```python
from build123d import *

# Parameters (mm, degrees)
SKETCH1_W           = 100
SKETCH1_H           = 105
SKETCH1_R           = 1.1
BOSS_EXTRUDE1_DEPTH = 2.5
SKETCH3_R           = 4
SKETCH3_R_2         = 1.1
BOSS_EXTRUDE2_DEPTH = 2.5
CHAMFER1_SIZE       = 1.25
SKETCH2_R           = 4.6
CUT_EXTRUDE1_DEPTH  = 0.6
SKETCH11_W          = 2.5
SKETCH11_H          = 2.5
BOSS_EXTRUDE5_DEPTH = 2.5


with BuildPart() as part:
    # Sketch1 → Boss-Extrude1 (new body)
    with BuildSketch(Plane(origin=(0, 0, 0), x_dir=(1, 0, 0), z_dir=(0, 1, 0))):
        Rectangle(SKETCH1_W, SKETCH1_H)
        with Locations(Location((-45, 45, 0), (0, 0, 270))):
            Circle(SKETCH1_R, mode=Mode.SUBTRACT)
        with Locations(Location((45, 45, 0), (0, 0, 90))):
            Circle(SKETCH1_R, mode=Mode.SUBTRACT)
        with Locations(Location((45, -45, 0), (0, 0, 270))):
            Circle(SKETCH1_R, mode=Mode.SUBTRACT)
        with Locations(Location((-45, -45, 0), (0, 0, 90))):
            Circle(SKETCH1_R, mode=Mode.SUBTRACT)
        Polygon((-40, 47.5), (40, 47.5), (40, 40), (47.5, 40), (47.5, -40), (40, -40), (40, -47.5), (-40, -47.5), (-40, -40), (-47.5, -40), (-47.5, 40), (-40, 40), align=None, mode=Mode.SUBTRACT)
    extrude(amount=BOSS_EXTRUDE1_DEPTH)

    # Sketch3 → Boss-Extrude2 (add)
    with BuildSketch(Plane(origin=(0, 0, 0), x_dir=(1, 0, 0), z_dir=(0, 1, 0))):
        with BuildLine():
            Line((-42.828427125, 40), (-6.891439137, 4.063012013))
            ThreePointArc((-6.891439137, 4.063012013), (-7.39103626, 3.061467459), (-7.745966692, 2))
            Line((-7.745966692, 2), (-40.338668084, 2))
            Line((-40.338668084, 2), (-47.5, 2))
            Line((-47.5, 2), (-47.5, -2))
            Line((-47.5, -2), (-43.661317629, -2))
            Line((-43.661317629, -2), (-7.745966692, -2))
            ThreePointArc((-7.745966692, -2), (-7.39103626, -3.061467459), (-6.891439137, -4.063012013))
            Line((-6.891439137, -4.063012013), (-42.828427125, -40))
            Line((-42.828427125, -40), (-40, -42.828427125))
            Line((-40, -42.828427125), (-4.063012013, -6.891439137))
            ThreePointArc((-4.063012013, -6.891439137), (-3.061467459, -7.39103626), (-2, -7.745966692))
            Line((-2, -7.745966692), (-2, -43.661317629))
            Line((-2, -43.661317629), (-2, -47.5))
            Line((-2, -47.5), (2, -47.5))
            Line((2, -47.5), (2, -43.661317629))
            Line((2, -43.661317629), (2, -7.745966692))
            ThreePointArc((2, -7.745966692), (3.061467459, -7.39103626), (4.063012013, -6.891439137))
            Line((4.063012013, -6.891439137), (40, -42.828427125))
            Line((40, -42.828427125), (42.828427125, -40))
            Line((42.828427125, -40), (6.891439137, -4.063012013))
            ThreePointArc((6.891439137, -4.063012013), (7.39103626, -3.061467459), (7.745966692, -2))
            Line((7.745966692, -2), (40.338675227, -2))
            ThreePointArc((40.338675227, -2), (42, -2.6), (43.661324773, -2))
            Line((43.661324773, -2), (47.5, -2))
            Line((47.5, -2), (47.5, 2))
            Line((47.5, 2), (43.661324773, 2))
            ThreePointArc((43.661324773, 2), (42, 2.6), (40.338675227, 2))
            Line((40.338675227, 2), (7.745966692, 2))
            ThreePointArc((7.745966692, 2), (7.39103626, 3.061467459), (6.891439137, 4.063012013))
            Line((6.891439137, 4.063012013), (42.828427125, 40))
            Line((42.828427125, 40), (40, 42.828427125))
            Line((40, 42.828427125), (4.063012013, 6.891439137))
            ThreePointArc((4.063012013, 6.891439137), (3.061467459, 7.39103626), (2, 7.745966692))
            Line((2, 7.745966692), (2, 40.338675227))
            ThreePointArc((2, 40.338675227), (2.6, 42), (2, 43.661324773))
            Line((2, 43.661324773), (2, 47.5))
            Line((2, 47.5), (-2, 47.5))
            Line((-2, 47.5), (-2, 43.661324773))
            ThreePointArc((-2, 43.661324773), (-2.6, 42), (-2, 40.338675227))
            Line((-2, 40.338675227), (-2, 7.745966692))
            ThreePointArc((-2, 7.745966692), (-3.061467459, 7.39103626), (-4.063012013, 6.891439137))
            Line((-4.063012013, 6.891439137), (-40, 42.828427125))
            Line((-40, 42.828427125), (-42.828427125, 40))
        make_face()
        with Locations(Location((0, 0, 0), (0, 0, 270))):
            Circle(SKETCH3_R, mode=Mode.SUBTRACT)
        with Locations(Location((0, 42, 0), (0, 0, 270))):
            Circle(SKETCH3_R_2, mode=Mode.SUBTRACT)
        with Locations(Location((42, 0, 0), (0, 0, 270))):
            Circle(SKETCH3_R_2, mode=Mode.SUBTRACT)
    extrude(amount=BOSS_EXTRUDE2_DEPTH)

    # Chamfer1
    chamfer1_edges = [part.edges().sort_by_distance(p)[0] for p in [
        (42, 2.5, -1.1),
        (-45, 2.5, -46.1),
        (45, 2.5, -43.9),
        (45, 2.5, 43.9),
        (-45, 2.5, 46.1),
        (0, 2.5, -43.1),
    ]]
    chamfer(chamfer1_edges, length=CHAMFER1_SIZE)

    # Sketch2 → Cut-Extrude1 (cut)
    with BuildSketch(Plane(origin=(0, 2.5, 0), x_dir=(1, 0, 0), z_dir=(0, 1, 0))):
        with Locations(Location((0, 0, 0), (0, 0, 270))):
            Circle(SKETCH2_R)
    extrude(amount=-CUT_EXTRUDE1_DEPTH, mode=Mode.SUBTRACT)

    # Sketch11 → Boss-Extrude5 (add)
    with BuildSketch(Plane(origin=(0, 2.5, 0), x_dir=(1, 0, 0), z_dir=(0, 1, 0))):
        with Locations((-51.25, 51.25)):
            Rectangle(SKETCH11_W, SKETCH11_H)
        with Locations((51.25, 51.25)):
            Rectangle(SKETCH11_W, SKETCH11_H)
        with Locations((-51.25, -51.25)):
            Rectangle(SKETCH11_W, SKETCH11_H)
        with Locations((51.25, -51.25)):
            Rectangle(SKETCH11_W, SKETCH11_H)
    extrude(amount=-BOSS_EXTRUDE5_DEPTH)


solid = part.part
```
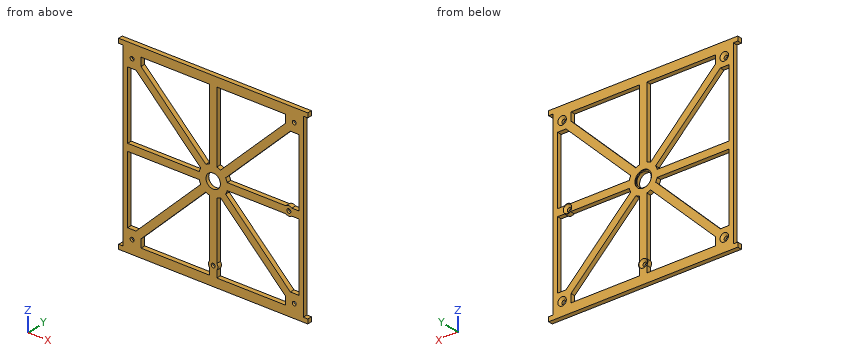
Design review of the part built by this model. Coordinates are the model's own, in mm. Coordinates: 2 decimals unless noted, no trailing zeros. Loops run counter-clockwise (first coordinate to the right, second up) from the corner with the lowest first, then second, coordinate; pieces in that order, holes last. Notation, with made-up numbers: M -28,68 L 6,68 A22 ccw 6,87 Z; hole C 33,13 d3. An arc over 180 degrees is marked long. One line per question, with ' | ' between items.
(1) We need section A-A (z = -10). Give the boundary of the cut face in (x, y).
Filled in:
outline: M -50,0 L -47.5,0 L -47.5,2.5 L -50,2.5 Z; M -12.83,0 L -7.17,0 L -7.17,2.5 L -12.83,2.5 Z; M -2,0 L 2,0 L 2,2.5 L -2,2.5 Z; M 7.17,0 L 12.83,0 L 12.83,2.5 L 7.17,2.5 Z; M 47.5,0 L 50,0 L 50,2.5 L 47.5,2.5 Z
(2) We need section C-C (y = 0.8). Count the separate pieces of the cut face and the enclosed holes in it, and give its area (3 significant figures).
Filled in:
separate pieces: 1 | enclosed holes: 15 | area: 3,290 mm^2
(3) Wall thickness on probe 1 along Z at (x, y) = (-43, 1.8); probe 2 along X at (y, z) = (0.3, -45); probe 3 along X at (y, z) = (1.25, -22.5): over which ranges is each line inside the solid? List them lowest first.
Filled in:
probe 1: z = -52.5 to -40, -2 to 2, 40 to 52.5 | probe 2: x = -50 to -46.1, -43.9 to -40, -2 to 2, 40 to 43.9, 46.1 to 50 | probe 3: x = -50 to -47.5, -25.33 to -19.67, -2 to 2, 19.67 to 25.33, 47.5 to 50
(4) For pin 1 Ø10 at (x, z) = (-21.5, 34) entering from +Y; pin 2 Ø0.8 at (y, z) = (1, -45) entering from +X, all flat-tipped, find the tip position at first contact; note any pin that passes through.
Filled in:
pin 1: passes through | pin 2: stops at x = 50
(5) We need section B-B (x = -38.5). Give the boundary of the cut face in (y, z), and give its area (3 significant figures).
Filled in:
outline: M 0,-52.5 L 2.5,-52.5 L 2.5,-47.5 L 0,-47.5 Z; M 0,-41.33 L 2.5,-41.33 L 2.5,-35.67 L 0,-35.67 Z; M 0,-2 L 2.5,-2 L 2.5,2 L 0,2 Z; M 0,35.67 L 2.5,35.67 L 2.5,41.33 L 0,41.33 Z; M 0,47.5 L 2.5,47.5 L 2.5,52.5 L 0,52.5 Z | area: 63.3 mm^2
